Here's how the part is built. I have some questions about the finished solid (model axes, mm). Face numbers are marked on the shaded views. A direction names the side the tool comes from. Give positions to 0.01 mm unless a question says otherwise; leave off trailing zeros. Write each loop counter-clockwise with the first axis right and the second up, starting at its lowest first coordinate (ties: lowest second). Pieces come first, ordered by that corner, then holes. Notation, with made-up numbers: (9.25, -30) -> (19.25, -30) arc R11 ccw to (19.25, -25) -> close; hole circle Ø7 at (85.5, 55.25). An arc over 180 degrees is marked (long way). Use CSV: the item, a comma, the result in double quotes. Start each with the question number.
(1) For pin 1 Ø7.5 at (x, y) = (-3.5, -2) entering from +Z; pin 2 Ø8 at (x, y) = (-8, 1.5) entering from +Z; pin 3 Ø3.5 at (x, y) = (-9.5, -2) entering from +Z, each with a flat end and sliding along its axis, tell me the tip position at first contact or that it passes through.
(2) I need wall thicknesses on L1, parallel to X at y = 5, z = 1.65; L2, parallel to X at y = 5, z = 0.9; L3, parallel to Y at x = -2, z = 1.95. Which ranges of each line are inside material? Lowest first, please. Write a range as [from, to].
(3) Suppose I cut it at C-C on x = -10.5. List the corners of the cut face in (y, z) for me.
(4) Suppose I cut it at B-B on y = -3.75. List the corners of the cut face in (x, z) for me.
(5) Which directions (+Z, -Z, +X, -X, +Y, -Y) give clear straight access to the entire face, cutting with the end or side of a thin tool? Please do the marked faces 1 and 2.
(6) Suppose I cut it at A-A on x = 2. List the corners of the cut face in (y, z) for me, plus the area to 3 significant figures.
(7) If we mould it in two halves opening along X, with no side actions, what happens to the marked faces 3, 4, 5 and 6? For each: pulls with the +X half, pulls with the -X half, needs draft (parallel to the pull), parting line crosses it, or undercut.
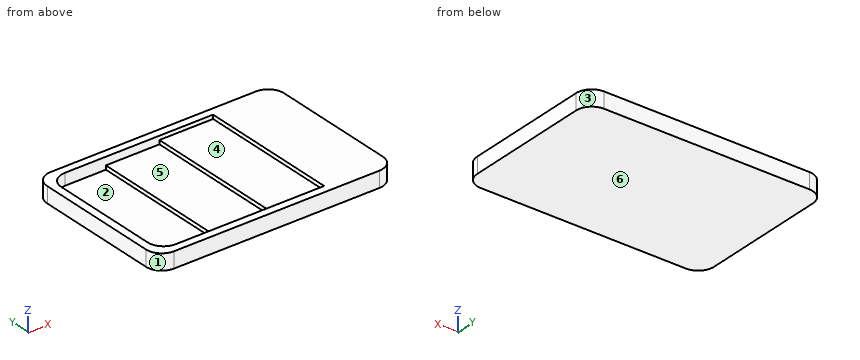
from build123d import *

# Parameters (mm, degrees)
F1_DEPTH = 2
F2_DEPTH = 0.5
F0_W     = 6.791314
F0_H     = 18
F3_DEPTH = 1.5
F4_DEPTH = 1
F5_DEPTH = 2


with BuildPart() as f1:
    # F0 (on Top) → F1 (new body)
    with BuildSketch(Plane.XY):
        with BuildLine():
            ThreePointArc((-15, -8), (-14.414214, -9.414214), (-13, -10))
            Line((-13, -10), (13, -10))
            ThreePointArc((13, -10), (14.414214, -9.414214), (15, -8))
            Line((15, -8), (15, 8))
            ThreePointArc((15, 8), (14.414214, 9.414214), (13, 10))
            Line((13, 10), (-13, 10))
            ThreePointArc((-13, 10), (-14.414214, 9.414214), (-15, 8))
            Line((-15, 8), (-15, -8))
        make_face()
        with BuildLine():
            ThreePointArc((-14, 7), (-13.414214, 8.414214), (-12, 9))
            Line((-12, 9), (-6.791314, 9))
            Line((-6.791314, 9), (0, 9))
            Line((0, 9), (6.791314, 9))
            Line((6.791314, 9), (12, 9))
            ThreePointArc((12, 9), (13.414214, 8.414214), (14, 7))
            Line((14, 7), (14, -7))
            ThreePointArc((14, -7), (13.414214, -8.414214), (12, -9))
            Line((12, -9), (6.791314, -9))
            Line((6.791314, -9), (0, -9))
            Line((0, -9), (-6.791314, -9))
            Line((-6.791314, -9), (-12, -9))
            ThreePointArc((-12, -9), (-13.414214, -8.414214), (-14, -7))
            Line((-14, -7), (-14, 7))
        make_face(mode=Mode.SUBTRACT)
    extrude(amount=F1_DEPTH)

    # F0 (on Top) → F2 (join)
    with BuildSketch(Plane.XY):
        with BuildLine():
            Line((-6.791314, 9), (-12, 9))
            ThreePointArc((-12, 9), (-13.414214, 8.414214), (-14, 7))
            Line((-14, 7), (-14, -7))
            ThreePointArc((-14, -7), (-13.414214, -8.414214), (-12, -9))
            Line((-12, -9), (-6.791314, -9))
            Line((-6.791314, -9), (-6.791314, 9))
        make_face()
    extrude(amount=F2_DEPTH)

    # F0 (on Top) → F3 (join)
    with BuildSketch(Plane.XY):
        with Locations((3.395657, 0)):
            Rectangle(F0_W, F0_H)
    extrude(amount=F3_DEPTH)

    # F0 (on Top) → F4 (join)
    with BuildSketch(Plane.XY):
        with Locations((-3.395657, 0)):
            Rectangle(F0_W, F0_H)
    extrude(amount=F4_DEPTH)

    # F0 (on Top) → F5 (join)
    with BuildSketch(Plane.XY):
        with BuildLine():
            Line((12, 9), (6.791314, 9))
            Line((6.791314, 9), (6.791314, -9))
            Line((6.791314, -9), (12, -9))
            ThreePointArc((12, -9), (13.414214, -8.414214), (14, -7))
            Line((14, -7), (14, 7))
            ThreePointArc((14, 7), (13.414214, 8.414214), (12, 9))
        make_face()
    extrude(amount=F5_DEPTH)


solid = f1.part
Geometry says:
1,pin 1,"z = 1.5"
1,pin 2,"z = 1"
1,pin 3,"z = 0.5"
2,L1,"[-15, -14], [6.79, 15]"
2,L2,"[-15, -14], [-6.79, 15]"
2,L3,"[-10, -9], [9, 10]"
3,outline,"(-10, 0) -> (10, 0) -> (10, 2) -> (9, 2) -> (9, 0.5) -> (-9, 0.5) -> (-9, 2) -> (-10, 2) -> close"
4,outline,"(-15, 0) -> (15, 0) -> (15, 2) -> (6.79, 2) -> (6.79, 1.5) -> (0, 1.5) -> (0, 1) -> (-6.79, 1) -> (-6.79, 0.5) -> (-14, 0.5) -> (-14, 2) -> (-15, 2) -> close"
5,face 1,"+Z, -Z, -X, -Y"
5,face 2,"+Z"
6,outline,"(-10, 0) -> (10, 0) -> (10, 2) -> (9, 2) -> (9, 1.5) -> (-9, 1.5) -> (-9, 2) -> (-10, 2) -> close"
6,area,"31.0 mm²"
7,face 3,"pulls with the +X half"
7,face 4,"undercut"
7,face 5,"undercut"
7,face 6,"needs draft"
